Here's how the part is built. I have some questions about the finished solid (model axes, mm). Face numbers are marked on the shaded views. A direction names the side the tool comes from. Round coordinates to 2 decimals unless told otherwise and drop trailing zeros. Order: outer loops, then holes, each group sorted by start corner. A loop starts at its lowest first (then second) coordinate and runs counter-clockwise, first axis right, second up. Notation, with made-up numbers: M 37,56.5 L 53,56.5 A15 ccw 53,63.5 Z; hole C 83.25,-10 d4. An arc over 180 degrees is marked long. Use one line per item in the form item = value. Start each with the question number.
Autodesk Inventor part; units mm, degrees
ref_plane "YZ Plane" through (0, 0, 0) normal (1, 0, 0) x (0, 1, 0)
ref_plane "XZ Plane" through (0, 0, 0) normal (0, 1, 0) x (-1, 0, 0)
ref_plane "XY Plane" through (0, 0, 0) normal (0, 0, 1) x (1, 0, 0)
sketch "Skizze1" plane through (0, 0, 0) normal (0, 0, 1) x (1, 0, 0)
  line L0 (0, 0) -> (-62, 0)
  line L1 (-62, 0) -> (-62, 23)
  line L2 (-62, 23) -> (0, 23)
  line L3 (0, 23) -> (0, 0)
  dimension "d0" = 62
  dimension "d1" = 23
extrude "Extrusion1" add sketch "Skizze1" along normal blind 96.5
sketch "Skizze2" plane through (-62, 23, 0) normal (0, 1, 0) x (1, 0, 0)
  circle A0 centre (31, -78.5) radius 7.0477
  line L0 (62, -96.5) -> (0, -96.5)
  line L1 (0, 0) -> (0, -96.5)
  point P0 (62, 0)
  dimension "d4" = 18
  dimension "d5" = 31
extrude "Extrusion2" cut sketch "Skizze2" against normal blind 10
fillet "Rundung1" radius 8 8 edges at (0, 23, 48.25) (0, 0, 48.25) (-62, 23, 48.25) (-62, 0, 48.25) (-31, 0, 96.5) (-31, 23, 96.5) (-31, 23, 0) (-31, 0, 0)
sketch "Skizze3" plane through (0, 0, 96.5) normal (0, 0, 1) x (1, 0, 0)
  line L0 (0, 8) -> (-62, 8)
  line L1 (0, 8) -> (0, 15)
  line L2 (-62, 15) -> (0, 15)
  line L3 (-62, 15) -> (-62, 8)
  line L4 (-57.1154, 17.1012) -> (-5.8036, 17.1012)
  line L5 (-5.8036, 17.1012) -> (-5.8036, 6.3302)
  line L6 (-5.8036, 6.3302) -> (-57.1154, 6.3302)
  line L7 (-57.1154, 6.3302) -> (-57.1154, 17.1012)
  point P0 (0, 0)
extrude "Extrusion3" cut sketch "Skizze3" against normal blind 10 contours L5 L6 L7 L0 | L0 L7 L2 L5 | L2 L7 L4 L5
properties part number "Anker"
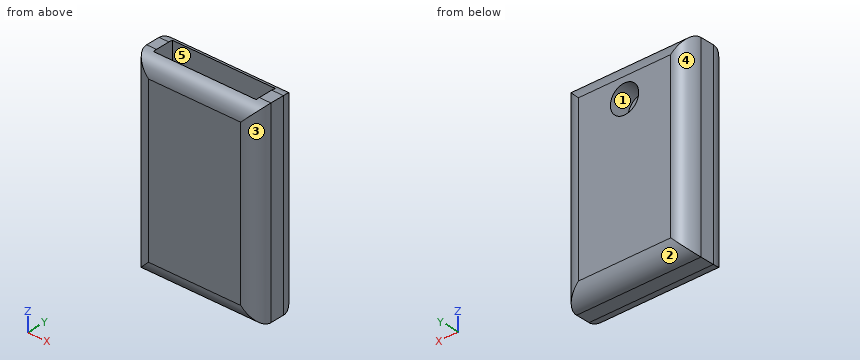
1) If I drill on line 1 (Z direction, x = -31, y = 20.5); line 2 (X direction, y = 18, z = 78.5); line 3 (X direction, y = 17.75, z = 78.5), over which ranges is the centre line in solid material (lowest first)?
2) If we section it at C-C on y = 20.25: Write out the boundary of the cut face in (x, z), then the cut area to 3 significant figures.
3) On a 3-axis mill with a long thin cutter (end or side, diameter ignored), from which of +Z, -Z, +X, -X, +Y, -Y can I reach the whole of each face in a straight line? I mean the marked faces 4 and 5. Say none if no direction works.
4) If we mould it in two halves opening along X, with no side actions, what happens to the marked faces 1, 2 and 3? For each: +X half, -X half, draft (parallel to the pull), parting line (faces both ways), or undercut.
5) If we section it at B-B on z = 78.5: Write out the boundary of the cut face in (x, y), then the cut area to 3 significant figures.
6) If we section it at A-A on x = -42.5: Write out the boundary of the cut face in (y, z), then the cut area to 3 significant figures.
7) Will these pins go through, and if not, where does the flat tip stop? pin 1 Ø8.5 at (x, y) = (-36, 9) entering from +Z; pin 2 Ø5 at (y, z) = (4, 15) entering from +X; pin 3 Ø4 at (x, z) = (-34.5, 77.5) entering from +Y.
8) If we section it at D-D on z = 67.5: Write out the boundary of the cut face in (x, y).
Completed:
q1.line_1 = 2.19 to 71.45, 85.55 to 94.31
q1.line_2 = -61.42 to -38.05, -23.95 to -0.58
q1.line_3 = -61.51 to -38.05, -23.95 to -0.49
q2.outline = M -60.04,1.96 L -1.96,1.96 L -1.96,94.54 L -60.04,94.54 Z; hole C -31,78.5 d14.1
q2.area = 5,220 mm²
q3.face_4 = +Z, -Z, -X, +Y
q3.face_5 = +Z
q4.face_1 = undercut
q4.face_2 = draft
q4.face_3 = +X half
q5.outline = M -62,8 A8 ccw -54,0 L -8,0 A8 ccw 0,8 L 0,15 A8 ccw -8,23 L -23.95,23 L -23.95,13 L -38.05,13 L -38.05,23 L -54,23 A8 ccw -62,15 Z
q5.area = 1,230 mm²
q6.outline = M 0,8 A8 ccw 8,0 L 15,0 A8 ccw 23,8 L 23,88.5 A8 ccw 17.1,96.22 L 17.1,86.5 L 6.33,86.5 L 6.33,96.32 A8 ccw 0,88.5 Z
q6.area = 2,060 mm²
q7.pin_1 = 96.32
q7.pin_2 = -0.14
q7.pin_3 = 13
q8.outline = M -62,8 A8 ccw -54,0 L -8,0 A8 ccw 0,8 L 0,15 A8 ccw -8,23 L -54,23 A8 ccw -62,15 Z
